Design review of the part shown in the three views and the two pictorial views. Dimensions are in mm from the part's minimum x, y and z. A direction names the side the tool comes from. Coordinates: 2 decimals unless noted, no trailing zeros. Loops run counter-clockwise (first coordinate to the right, second up) from the corner with the lowest first, then second, coordinate; pieces in that order, holes last. Notation, with made-up numbers: (77, -24.75) -> (133, -24.75) arc R26 cw to (133, 1.25) -> close; hole circle Ø3 at (-1, -22). An arc over 180 degrees is marked (long way). Answer in a Markdown table with one row per item.
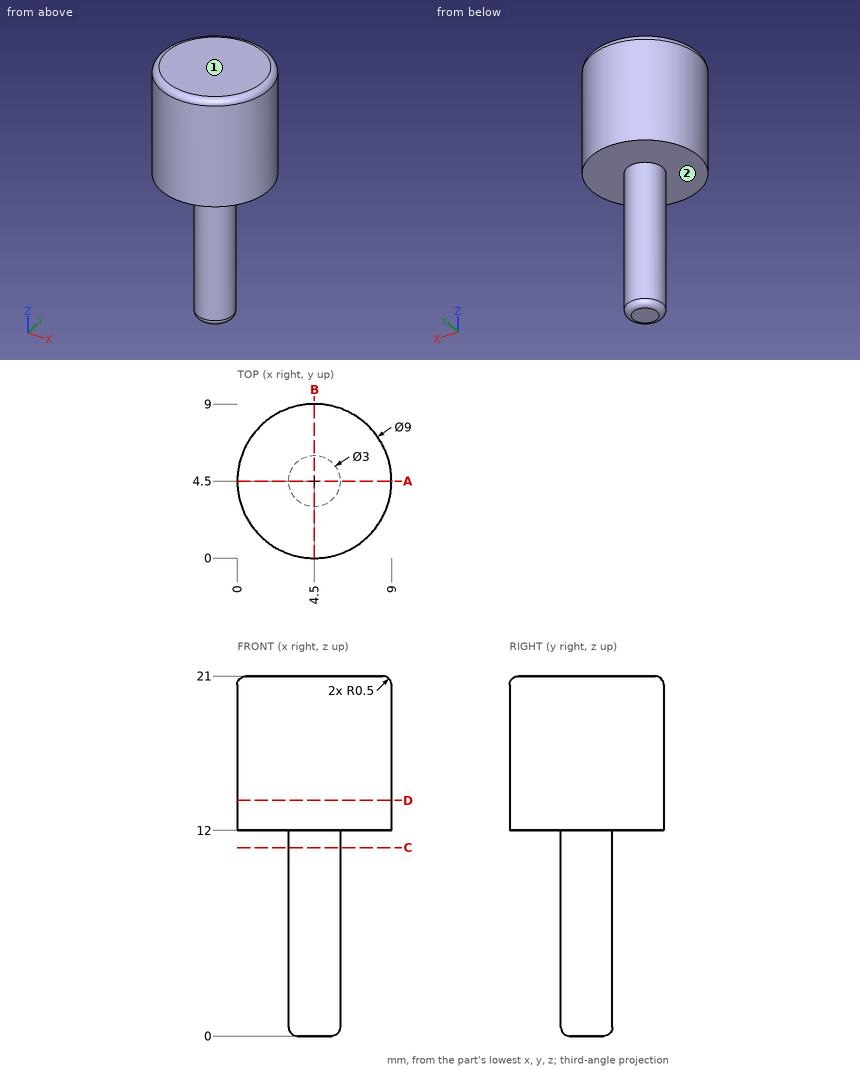
(1) To check wall thickness, follow probe 1 along Z at (x, y) = (6, 4); probe 2 along X at (y, z) = (5.75, 6.75); probe 3 along X at (y, z) = (7.75, 17.75). State the ranges of each line that lie inside material, in increasing order.
Evaluation:
| item | result |
|---|---|
| probe 1 | z = 12 to 21 |
| probe 2 | x = 3.67 to 5.33 |
| probe 3 | x = 1.39 to 7.61 |
(2) Take a section at C-C on z = 11. Give the boundary of the cut face in (x, y), and give its area (3 significant figures).
Evaluation:
| item | result |
|---|---|
| outline | circle Ø3 at (4.5, 4.5) |
| area | 7.07 mm² |
(3) Take a section at A-A on y = 4.5. Give the boundary of the cut face in (x, z).
Evaluation:
| item | result |
|---|---|
| outline | (0, 12) -> (3, 12) -> (3, 0.5) arc R0.5 ccw to (3.5, 0) -> (5.5, 0) arc R0.5 ccw to (6, 0.5) -> (6, 12) -> (9, 12) -> (9, 20.5) arc R0.5 ccw to (8.5, 21) -> (0.5, 21) arc R0.5 ccw to (0, 20.5) -> close |
(4) Take a section at D-D on z = 13.75. Give the boundary of the cut face in (x, y), and give its area (3 significant figures).
Evaluation:
| item | result |
|---|---|
| outline | circle Ø9 at (4.5, 4.5) |
| area | 63.6 mm² |
(5) Tool access review of the marked faces 1 and 2: name each direction out of +Z, -Z, +X, -X, +Y, -Y from which nothing blocks a thin tool from reaching the whole face with its end or side.
Evaluation:
| item | result |
|---|---|
| face 1 | +Z, +X, -X, +Y, -Y |
| face 2 | -Z |
(6) For pin 1 (4 mm diameter, centred on x = 8, z = 11, fed in from -Y); pin 2 (5 mm diameter, centred on x = 7, z = 8.5, fed in from -Y); pin 3 (3 mm diameter, centred on x = 2, z = 3.5, fed in from -Y), all flat-tipped, find the tip position at first contact; note any pin that passes through.
Evaluation:
| item | result |
|---|---|
| pin 1 | stops at y = 0.36 |
| pin 2 | stops at y = 3 |
| pin 3 | stops at y = 3.38 |
